```python
from build123d import *

# Parameters (mm, degrees)
SKETCH_1_W          = 44.2
SKETCH_1_H          = 20
EXTRUDE_1_DEPTH     = 2
CUT_EXTRUDE_1_REACH = 4
SKETCH_2_R          = 3
SKETCH_2_R_2        = 1.5
SKETCH_3_W          = 20
SKETCH_3_H          = 25
EXTRUDE_2_DEPTH     = 2
CUT_EXTRUDE_2_REACH = 46.2
SKETCH_4_R          = 4
SKETCH_4_R_2        = 1
CUT_EXTRUDE_3_REACH = 46.2
SKETCH_5_R          = 4
SKETCH_5_R_2        = 1


with BuildPart() as part:
    # 草图1 → 凸台-拉伸1 (new body)
    with BuildSketch(Plane(origin=(0, 0, 0), x_dir=(1, 0, 0), z_dir=(0, 1, 0))):
        Rectangle(SKETCH_1_W, SKETCH_1_H)
    extrude(amount=EXTRUDE_1_DEPTH)

    # 草图2 → 切除-拉伸1 (cut, up to next)
    with BuildSketch(Plane(origin=(0, 2, 0), x_dir=(1, 0, 0), z_dir=(0, 1, 0)), mode=Mode.PRIVATE) as cut_extrude_1_sk1:
        Circle(SKETCH_2_R)
    cut_extrude_1_tool1 = extrude(cut_extrude_1_sk1.sketch, amount=-CUT_EXTRUDE_1_REACH, mode=Mode.PRIVATE) & part.part
    add(cut_extrude_1_tool1.solids().sort_by_distance((0, 2, 0))[0], mode=Mode.SUBTRACT)
    # 草图2 → 切除-拉伸1 (cut, up to next)
    with BuildSketch(Plane(origin=(0, 2, 0), x_dir=(1, 0, 0), z_dir=(0, 1, 0)), mode=Mode.PRIVATE) as cut_extrude_1_sk2:
        with Locations((4.949747468, -4.949747468)):
            Circle(SKETCH_2_R_2)
    cut_extrude_1_tool2 = extrude(cut_extrude_1_sk2.sketch, amount=-CUT_EXTRUDE_1_REACH, mode=Mode.PRIVATE) & part.part
    add(cut_extrude_1_tool2.solids().sort_by_distance((4.949747, 2, 4.949747))[0], mode=Mode.SUBTRACT)
    # 草图2 → 切除-拉伸1 (cut, up to next)
    with BuildSketch(Plane(origin=(0, 2, 0), x_dir=(1, 0, 0), z_dir=(0, 1, 0)), mode=Mode.PRIVATE) as cut_extrude_1_sk3:
        with Locations((-4.949747468, -4.949747468)):
            Circle(SKETCH_2_R_2)
    cut_extrude_1_tool3 = extrude(cut_extrude_1_sk3.sketch, amount=-CUT_EXTRUDE_1_REACH, mode=Mode.PRIVATE) & part.part
    add(cut_extrude_1_tool3.solids().sort_by_distance((-4.949747, 2, 4.949747))[0], mode=Mode.SUBTRACT)
    # 草图2 → 切除-拉伸1 (cut, up to next)
    with BuildSketch(Plane(origin=(0, 2, 0), x_dir=(1, 0, 0), z_dir=(0, 1, 0)), mode=Mode.PRIVATE) as cut_extrude_1_sk4:
        with Locations((-4.949747468, 4.949747468)):
            Circle(SKETCH_2_R_2)
    cut_extrude_1_tool4 = extrude(cut_extrude_1_sk4.sketch, amount=-CUT_EXTRUDE_1_REACH, mode=Mode.PRIVATE) & part.part
    add(cut_extrude_1_tool4.solids().sort_by_distance((-4.949747, 2, -4.949747))[0], mode=Mode.SUBTRACT)
    # 草图2 → 切除-拉伸1 (cut, up to next)
    with BuildSketch(Plane(origin=(0, 2, 0), x_dir=(1, 0, 0), z_dir=(0, 1, 0)), mode=Mode.PRIVATE) as cut_extrude_1_sk5:
        with Locations((4.949747468, 4.949747468)):
            Circle(SKETCH_2_R_2)
    cut_extrude_1_tool5 = extrude(cut_extrude_1_sk5.sketch, amount=-CUT_EXTRUDE_1_REACH, mode=Mode.PRIVATE) & part.part
    add(cut_extrude_1_tool5.solids().sort_by_distance((4.949747, 2, -4.949747))[0], mode=Mode.SUBTRACT)

    # 草图3 → 凸台-拉伸2 (add)
    with BuildSketch(Plane.ZY.offset(22.1)):
        with Locations((0, 14.5)):
            Rectangle(SKETCH_3_W, SKETCH_3_H)
    extrude_2 = extrude(amount=-EXTRUDE_2_DEPTH)

    # 镜向2: 凸台-拉伸2 across plane
    add(extrude_2.mirror(Plane.ZY))

    # 草图4 → 切除-拉伸2 (cut, up to next)
    with BuildSketch(Plane.ZY.offset(22.1), mode=Mode.PRIVATE) as cut_extrude_2_sk1:
        with BuildLine():
            ThreePointArc((-10, 17), (-7.071067806, 24.071067818), (1.6e-08, 27))
            Line((1.6e-08, 27), (-10, 27))
            Line((-10, 27), (-10, 17))
        make_face()
    cut_extrude_2_tool1 = extrude(cut_extrude_2_sk1.sketch, amount=-CUT_EXTRUDE_2_REACH, mode=Mode.PRIVATE) & part.part
    add(cut_extrude_2_tool1.solids().sort_by_distance((-22.1, 24.766321, -7.766321))[0], mode=Mode.SUBTRACT)
    # 草图4 → 切除-拉伸2 (cut, up to next)
    with BuildSketch(Plane.ZY.offset(22.1), mode=Mode.PRIVATE) as cut_extrude_2_sk2:
        with BuildLine():
            Line((10, 17), (10, 27))
            Line((10, 27), (1.6e-08, 27))
            ThreePointArc((1.6e-08, 27), (7.071067818, 24.071067806), (10, 17))
        make_face()
    cut_extrude_2_tool2 = extrude(cut_extrude_2_sk2.sketch, amount=-CUT_EXTRUDE_2_REACH, mode=Mode.PRIVATE) & part.part
    add(cut_extrude_2_tool2.solids().sort_by_distance((-22.1, 24.766321, 7.766321))[0], mode=Mode.SUBTRACT)
    # 草图4 → 切除-拉伸2 (cut, up to next)
    with BuildSketch(Plane.ZY.offset(22.1), mode=Mode.PRIVATE) as cut_extrude_2_sk3:
        with Locations((0, 17)):
            Circle(SKETCH_4_R)
    cut_extrude_2_tool3 = extrude(cut_extrude_2_sk3.sketch, amount=-CUT_EXTRUDE_2_REACH, mode=Mode.PRIVATE) & part.part
    add(cut_extrude_2_tool3.solids().sort_by_distance((-22.1, 17, 0))[0], mode=Mode.SUBTRACT)
    # 草图4 → 切除-拉伸2 (cut, up to next)
    with BuildSketch(Plane.ZY.offset(22.1), mode=Mode.PRIVATE) as cut_extrude_2_sk4:
        with Locations((0, 24)):
            Circle(SKETCH_4_R_2)
    cut_extrude_2_tool4 = extrude(cut_extrude_2_sk4.sketch, amount=-CUT_EXTRUDE_2_REACH, mode=Mode.PRIVATE) & part.part
    add(cut_extrude_2_tool4.solids().sort_by_distance((-22.1, 24, 0))[0], mode=Mode.SUBTRACT)
    # 草图4 → 切除-拉伸2 (cut, up to next)
    with BuildSketch(Plane.ZY.offset(22.1), mode=Mode.PRIVATE) as cut_extrude_2_sk5:
        with Locations((7, 17)):
            Circle(SKETCH_4_R_2)
    cut_extrude_2_tool5 = extrude(cut_extrude_2_sk5.sketch, amount=-CUT_EXTRUDE_2_REACH, mode=Mode.PRIVATE) & part.part
    add(cut_extrude_2_tool5.solids().sort_by_distance((-22.1, 17, 7))[0], mode=Mode.SUBTRACT)
    # 草图4 → 切除-拉伸2 (cut, up to next)
    with BuildSketch(Plane.ZY.offset(22.1), mode=Mode.PRIVATE) as cut_extrude_2_sk6:
        with Locations((0, 10)):
            Circle(SKETCH_4_R_2)
    cut_extrude_2_tool6 = extrude(cut_extrude_2_sk6.sketch, amount=-CUT_EXTRUDE_2_REACH, mode=Mode.PRIVATE) & part.part
    add(cut_extrude_2_tool6.solids().sort_by_distance((-22.1, 10, 0))[0], mode=Mode.SUBTRACT)
    # 草图4 → 切除-拉伸2 (cut, up to next)
    with BuildSketch(Plane.ZY.offset(22.1), mode=Mode.PRIVATE) as cut_extrude_2_sk7:
        with Locations((-7, 17)):
            Circle(SKETCH_4_R_2)
    cut_extrude_2_tool7 = extrude(cut_extrude_2_sk7.sketch, amount=-CUT_EXTRUDE_2_REACH, mode=Mode.PRIVATE) & part.part
    add(cut_extrude_2_tool7.solids().sort_by_distance((-22.1, 17, -7))[0], mode=Mode.SUBTRACT)

    # 草图5 → 切除-拉伸3 (cut, up to next)
    with BuildSketch(Plane(origin=(22.1, 0, 0), x_dir=(0, 0, -1), z_dir=(1, 0, 0)), mode=Mode.PRIVATE) as cut_extrude_3_sk1:
        with Locations((0, 17)):
            Circle(SKETCH_5_R)
    cut_extrude_3_tool1 = extrude(cut_extrude_3_sk1.sketch, amount=-CUT_EXTRUDE_3_REACH, mode=Mode.PRIVATE) & part.part
    add(cut_extrude_3_tool1.solids().sort_by_distance((22.1, 17, 0))[0], mode=Mode.SUBTRACT)
    # 草图5 → 切除-拉伸3 (cut, up to next)
    with BuildSketch(Plane(origin=(22.1, 0, 0), x_dir=(0, 0, -1), z_dir=(1, 0, 0)), mode=Mode.PRIVATE) as cut_extrude_3_sk2:
        with Locations((-7.5, 24.5)):
            Circle(SKETCH_5_R_2)
    cut_extrude_3_tool2 = extrude(cut_extrude_3_sk2.sketch, amount=-CUT_EXTRUDE_3_REACH, mode=Mode.PRIVATE) & part.part
    add(cut_extrude_3_tool2.solids().sort_by_distance((22.1, 24.5, 7.5))[0], mode=Mode.SUBTRACT)
    # 草图5 → 切除-拉伸3 (cut, up to next)
    with BuildSketch(Plane(origin=(22.1, 0, 0), x_dir=(0, 0, -1), z_dir=(1, 0, 0)), mode=Mode.PRIVATE) as cut_extrude_3_sk3:
        with Locations((7.5, 24.5)):
            Circle(SKETCH_5_R_2)
    cut_extrude_3_tool3 = extrude(cut_extrude_3_sk3.sketch, amount=-CUT_EXTRUDE_3_REACH, mode=Mode.PRIVATE) & part.part
    add(cut_extrude_3_tool3.solids().sort_by_distance((22.1, 24.5, -7.5))[0], mode=Mode.SUBTRACT)
    # 草图5 → 切除-拉伸3 (cut, up to next)
    with BuildSketch(Plane(origin=(22.1, 0, 0), x_dir=(0, 0, -1), z_dir=(1, 0, 0)), mode=Mode.PRIVATE) as cut_extrude_3_sk4:
        with Locations((7.5, 9.5)):
            Circle(SKETCH_5_R_2)
    cut_extrude_3_tool4 = extrude(cut_extrude_3_sk4.sketch, amount=-CUT_EXTRUDE_3_REACH, mode=Mode.PRIVATE) & part.part
    add(cut_extrude_3_tool4.solids().sort_by_distance((22.1, 9.5, -7.5))[0], mode=Mode.SUBTRACT)
    # 草图5 → 切除-拉伸3 (cut, up to next)
    with BuildSketch(Plane(origin=(22.1, 0, 0), x_dir=(0, 0, -1), z_dir=(1, 0, 0)), mode=Mode.PRIVATE) as cut_extrude_3_sk5:
        with Locations((-7.5, 9.5)):
            Circle(SKETCH_5_R_2)
    cut_extrude_3_tool5 = extrude(cut_extrude_3_sk5.sketch, amount=-CUT_EXTRUDE_3_REACH, mode=Mode.PRIVATE) & part.part
    add(cut_extrude_3_tool5.solids().sort_by_distance((22.1, 9.5, 7.5))[0], mode=Mode.SUBTRACT)


solid = part.part
```
Here's how the part is built. I have some questions about the finished solid (model axes, mm). A direction names the side the tool comes from. Give positions to 0.01 mm unless a question says otherwise; leave off trailing zeros. Loops run counter-clockwise (first coordinate to the right, second up) from the corner with the lowest first, then second, coordinate; pieces in that order, holes last. Notation, with made-up numbers: M 75,-1 L 83,-1 A32 ccw 83,36 Z; hole C 43.25,29 d7. An arc over 180 degrees is marked long. Put each result on its own line as item: value. Start each with the question number.
(1) I need wall thicknesses on line 1 along Y through (x, z) = (20.65, 7.5); line 2 along X through (y, z) = (8.25, 9); line 3 along X through (y, z) = (17.5, -7.5). Which ranges of each line are inside material? Lowest first, please. Write a range as [from, to].
(2) I want a section at C-C on z = 5.5. Please give me the cut outline in (x, y), then the cut area to 3 significant figures.
(3) I want a section at B-B on x = 0. Please give me the cut outline in (y, z), then the cut area to 3 significant figures.
(4) I want a section at D-D on z = -2.5. Please give me the cut outline in (x, y).
(5) For faces 5 (the cylindrical face through (21.114, 20.966, 0.521)), 6 (the flat face through (2, 1, -10)), 7 (the flat face through (-20.1, 12, 0)), 8 (the cylindrical face through (-21, 23, 0)), 9 (the cylindrical face through (21.114, 23.524, -7.283)), which set-ups out of +Z, -Z, +X, -X, +Y, -Y let a thin tool reach every point of the face, with its end or its side?
(6) If we mould it in two halves opening along X, with no side actions, what happens to faces 1 (the flat face through (22.1, 11, 0)), 2 (the cylindrical face through (5.756, 1.014, 3.685)), 3 (the cylindrical face through (6.335, 1.014, -4.375)), 4 (the cylindrical face through (-21, 11, 0))? For each: +X half, -X half, draft (parallel to the pull), parting line (faces both ways), or undercut.
(7) I want a section at A-A on y = 12. Please give me the cut outline in (x, z).
(8) Will these pins go through, and if not, where does the flat tip stop? pin 1 Ø5 at (x, z) = (4.95, -4.95) entering from +Y; pin 2 Ø1.8 at (y, z) = (24, 0) entering from -X.
Answer block:
1. line 1: [0, 8.5], [10.5, 23.5], [25.5, 27]
1. line 2: [-22.1, -20.1], [20.1, 22.1]
1. line 3: [20.1, 22.1]
2. outline: M -22.1,0 L -6.35,0 L -6.35,2 L -20.1,2 L -20.1,25.35 L -22.1,25.35 Z; M -3.55,0 L 3.55,0 L 3.55,2 L -3.55,2 Z; M 6.35,0 L 22.1,0 L 22.1,27 L 20.1,27 L 20.1,2 L 6.35,2 Z
2. area: 174 mm^2
3. outline: M 0,-10 L 2,-10 L 2,-3 L 0,-3 Z; M 0,3 L 2,3 L 2,10 L 0,10 Z
3. area: 28.0 mm^2
4. outline: M -22.1,0 L -1.66,0 L -1.66,2 L -20.1,2 L -20.1,13.88 L -22.1,13.88 Z; M -22.1,20.12 L -20.1,20.12 L -20.1,26.68 L -22.1,26.68 Z; M 1.66,0 L 22.1,0 L 22.1,13.88 L 20.1,13.88 L 20.1,2 L 1.66,2 Z; M 20.1,20.12 L 22.1,20.12 L 22.1,27 L 20.1,27 Z
5. face 5: +X, -X
5. face 6: -Z, +X, -X, +Y, -Y
5. face 7: +Z, -Z, +Y
5. face 8: -X
5. face 9: +X
6. face 1: +X half
6. face 2: undercut
6. face 3: undercut
6. face 4: draft
7. outline: M -22.1,-10 L -20.1,-10 L -20.1,10 L -22.1,10 Z; M 20.1,-10 L 22.1,-10 L 22.1,10 L 20.1,10 Z
8. pin 1: y = 2
8. pin 2: x = 20.1
